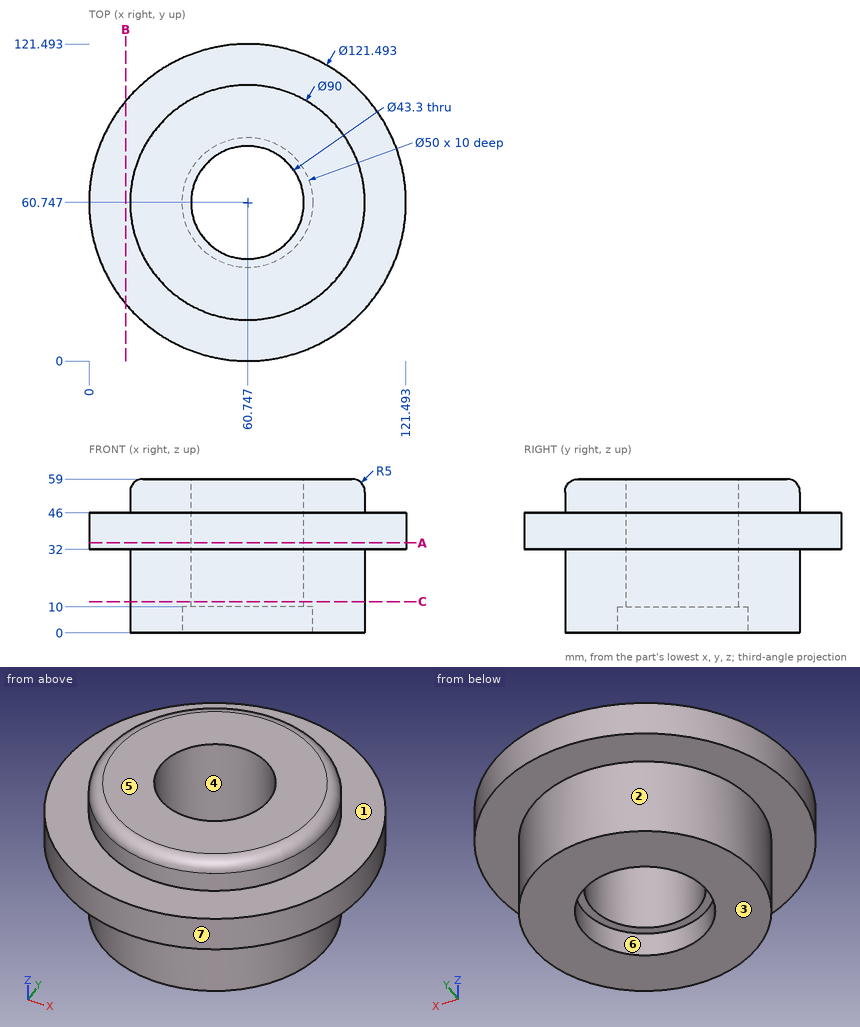
Input: dimensioned drawing with shaded views. Units: mm. Origin: part minimum x, y, z. A direction names the side the tool comes from. Give positions to 0.01 mm unless a question says otherwise; leave off trailing zeros. Loops run counter-clockwise (first coordinate to the right, second up) from the corner with the lowest first, then second, coordinate; pieces in that order, holes last. Notation, with made-up numbers: (87.5, 4.25) - (95.5, 4.25) arc R25 cw to (95.5, 40.25) - close; hole circle Ø7 at (-19, 9.25). An arc over 180 degrees is marked (long way). Answer as CSV lines item,"result". Start each with the question number.
(1) Section query C-C (z = 12). Output: boundary loops of the cut face in (x, y), and give its area (3 significant figures).
(2) Section query A-A (z = 34.5). Output: boundary loops of the cut face in (x, y).
(3) Mould query, pull axis Y, two halves, no side actions, for the marked faces 4, 5, 6 and 7. Classes: +Y half, -Y half, draft (parallel to the pull), parting line (faces both ways), or undercut.
(4) Reachability of the marked faces 1, 2 and 3 from +Z, -Z, +X, -X, +Y, -Y: full face, straight path, thin tool, end or side. Return the list, or none.
(5) Pin query (flat end, axial travel): P1, Ø1.5, axis at x = 94, y = 16.5, coming from the -Z side; P2, Ø1, axis at x = 53.5, z = 41.5, coming from the -Y side; P3, Ø8, axis at x = 34.5, z = 40.5, coming from the +Y side. Return the tip coordinate at first contact, or that it passes through.
(6) Ray query, line 1 along Z through (x, y) = (54.5, 9.5); line 2 along Y through (x, z) = (48.5, 39) (1 decimal); line 3 along X through (y, z) = (57, 29). Return the intervals inside material, ascending. Write a range as [from, to].
(7) Section query B-B (x = 14). Output: boundary loops of the cut face in (y, z).
Worked answers:
1,outline,"circle Ø90 at (60.75, 60.75); hole circle Ø43.3 at (60.75, 60.75)"
1,area,"4,890 mm^2"
2,outline,"circle Ø121.49 at (60.75, 60.75); hole circle Ø43.3 at (60.75, 60.75)"
3,face 4,"undercut"
3,face 5,"draft"
3,face 6,"undercut"
3,face 7,"parting line"
4,face 1,"+Z"
4,face 2,"-Z"
4,face 3,"-Z, +X, -X, +Y, -Y"
5,P1,"stops at z = 32"
5,P2,"stops at y = 0.38"
5,P3,"stops at y = 117.27"
6,line 1,"z = [32, 46]"
6,line 2,"y = [1.2, 42.9], [78.6, 120.2]"
6,line 3,"x = [15.9, 39.42], [82.07, 105.59]"
7,outline,"(21.95, 32) - (99.54, 32) - (99.54, 46) - (21.95, 46) - close"
